Answer from the drawing. Dimensions are ordinates in mm from the lowest x, y and z of the part. Coordinates: 2 decimals unless noted, no trailing zeros. Write each loop counter-clockwise with the first axis right and the second up, starting at its lowest first coordinate (ties: lowest second). Pieces come first, ordered by that corner, then holes. Notation, with made-up numbers: (26.5, 41) -> (37.5, 41) arc R27 cw to (37.5, 67) -> close; hole circle Ø4 at (-18.75, 17.25). An arc over 180 degrees is marked (long way). One line per item, written item: value. Start each with the question number.
1. Find section A-A, the plane y = 2.75. Write down the section's boundary in (x, z), and give its area (3 significant figures).
2. For a pull along Y with two mould halves and no side action, classify the marked faces 1, 2 and 3 as pulls with the +Y half, pulls with the -Y half, needs draft (parallel to the pull), parting line crosses it, or undercut.
3. Consider line 1 along X through (y, z) = (2.9, 7.25); line 2 along Y through (x, z) = (2.8, 7); line 3 along X through (y, z) = (2.75, 2). Determine where each line is inside the solid, lowest interval first.
4. Given P1, Ø2, axis at x = 10, z = 4, coming from the -Y side, flat-ended and moving along its own axis, determine where the tip first touches the part or whether it passes through.
5. Find section B-B, the plane x = 22.7. Write down the section's boundary in (y, z).
6. Find section D-D, the plane y = 4.7. Write down the section's boundary in (x, z), and give its area (3 significant figures).
7. Find section C-C, the plane z = 4.5. Write down the section's boundary in (x, y).
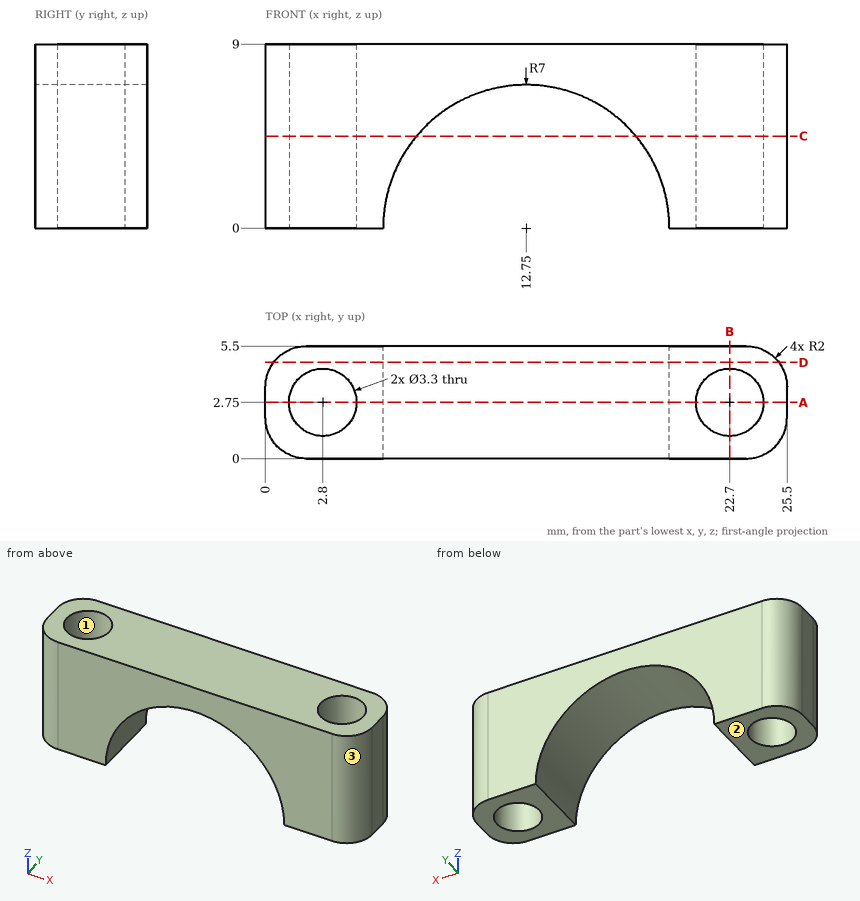
Answer block:
1. outline: (0, 0) -> (1.15, 0) -> (1.15, 9) -> (0, 9) -> close; (4.45, 0) -> (5.75, 0) arc R7 cw to (19.75, 0) -> (21.05, 0) -> (21.05, 9) -> (4.45, 9) -> close; (24.35, 0) -> (25.5, 0) -> (25.5, 9) -> (24.35, 9) -> close
1. area: 93.1 mm2
2. face 1: undercut
2. face 2: needs draft
2. face 3: pulls with the -Y half
3. line 1: x = 0 to 1.16, 4.44 to 21.06, 24.34 to 25.5
3. line 2: y = 0 to 1.1, 4.4 to 5.5
3. line 3: x = 0 to 1.15, 4.45 to 6.04, 19.46 to 21.05, 24.35 to 25.5
4. P1: passes through
5. outline: (0, 0) -> (1.1, 0) -> (1.1, 9) -> (0, 9) -> close; (4.4, 0) -> (5.5, 0) -> (5.5, 9) -> (4.4, 9) -> close
6. outline: (0.4, 0) -> (5.75, 0) arc R7 cw to (19.75, 0) -> (25.1, 0) -> (25.1, 9) -> (0.4, 9) -> close
6. area: 145 mm2
7. outline: (0, 2) arc R2 ccw to (2, 0) -> (7.39, 0) -> (7.39, 5.5) -> (2, 5.5) arc R2 ccw to (0, 3.5) -> close; (18.11, 0) -> (23.5, 0) arc R2 ccw to (25.5, 2) -> (25.5, 3.5) arc R2 ccw to (23.5, 5.5) -> (18.11, 5.5) -> close; hole circle Ø3.3 at (2.8, 2.75); hole circle Ø3.3 at (22.7, 2.75)
